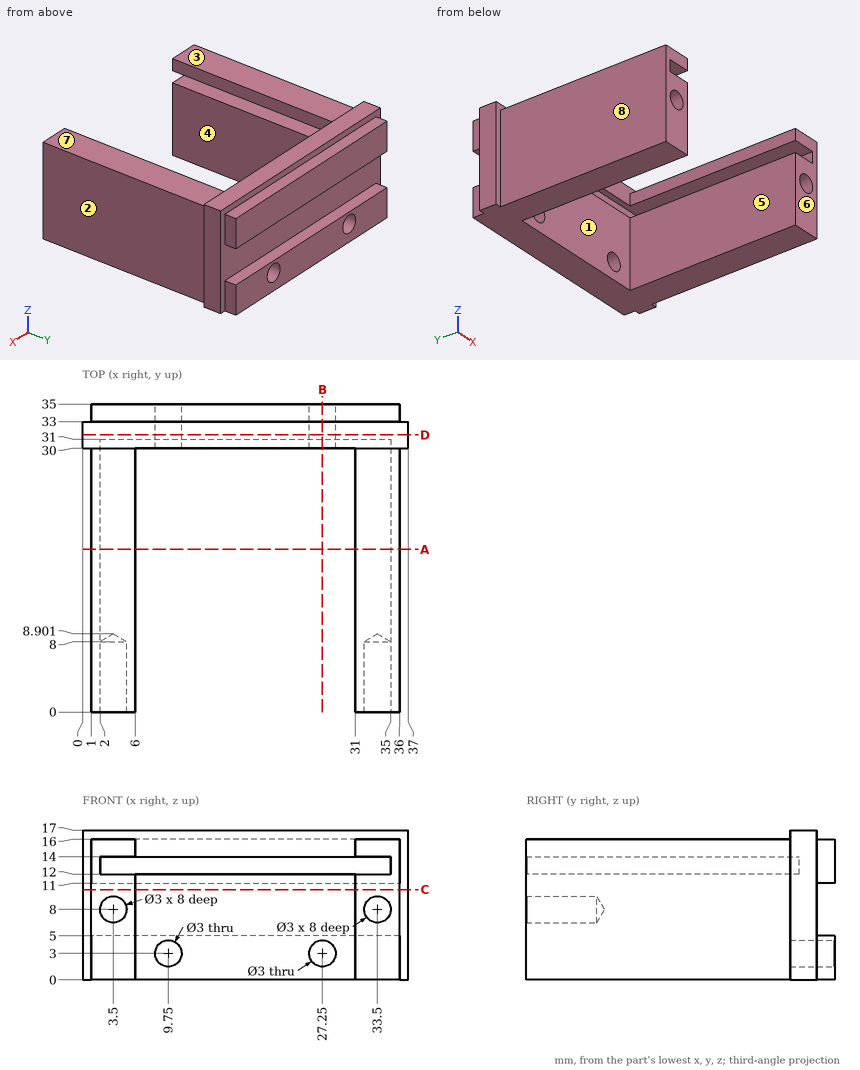
Job drawing, mm, ordinate dimensions from the low corner. One solid piece. A direction names the side the tool comes from. Give positions to 0.01 mm unless a question says otherwise; leave off trailing zeros. Write each loop counter-clockwise with the first axis right and the second up, starting at its lowest first coordinate (ties: lowest second). Pieces come first, ordered by that corner, then holes. Notation, with made-up numbers: (78.25, 28.5) - (116.25, 28.5) arc R16 cw to (116.25, 33.5) - close; hole circle Ø3 at (81.25, 54.5). An arc over 180 degrees is marked (long way). Use one line per item in the form item = value. Start each with the question number.
1. Two-plate mould, pull along X, no slides. Class the marked faces 1, 2, 3 and 4: released by +X, released by -X, zero draft, split by the parting line, or undercut.
2. Band-saw the part on D-D on y = 31.5. Write the cut outline in (x, z).
3. Drop flat-ended pins along their axis: pin 1 Ø1.6 at (y, z) = (34, 12.5) entering from -X; pin 2 Ø1.6 at (x, y) = (17, 34) entering from +Z; pin 3 Ø8 at (x, z) = (16, 14.5) entering from -Y; pin 4 Ø2 at (x, z) = (4, 14) entering from -Y. Give the stop position or say it passes through.
4. Band-saw the part on C-C on z = 10.25. Write the cut outline in (x, y), plus the area to 3 significant figures.
5. Probe line 1 (Z direction, x = 33.5, y = 5); line 2 (Z direction, x = 27.25, y = 33.2); line 3 (X direction, y = 32.2, z = 3). List the from-to ranges inside material, lowest first. Write a range as [from, to].
6. 3-axis set-ups, long thin cutter, end or side, ignore diameter. For the marked faces 5, 6, 7 and 8: which of +Z, -Z, +X, -X, +Y, -Y reach the whole face in a straight line?
7. Band-saw the part on A-A on y = 18.5. Write the cut outline in (x, z), plus the area to 3 significant figures.
8. Band-saw the part on B-B on x = 27.25. Write the cut outline in (y, z).
Conclusion:
q1.face_1 = undercut
q1.face_2 = released by +X
q1.face_3 = zero draft
q1.face_4 = undercut
q2.outline = (0, 0) - (37, 0) - (37, 17) - (0, 17) - close; hole circle Ø3 at (9.75, 3); hole circle Ø3 at (27.25, 3)
q3.pin_1 = 1
q3.pin_2 = 16
q3.pin_3 = 30
q3.pin_4 = 0
q4.outline = (0, 30) - (1, 30) - (1, 0) - (6, 0) - (6, 30) - (31, 30) - (31, 0) - (36, 0) - (36, 30) - (37, 30) - (37, 33) - (0, 33) - close
q4.area = 411 mm²
q5.line_1 = [0, 6.5], [9.5, 12], [14, 16]
q5.line_2 = [0, 1.5], [4.5, 5], [11, 16]
q5.line_3 = [0, 8.25], [11.25, 25.75], [28.75, 37]
q6.face_5 = +Z, -Z, -Y
q6.face_6 = +Z, -Z, +X, -X, -Y
q6.face_7 = +Z, +X, -X, -Y
q6.face_8 = +Z, -Z, -X, -Y
q7.outline = (1, 0) - (6, 0) - (6, 12) - (2, 12) - (2, 14) - (6, 14) - (6, 16) - (1, 16) - close; (31, 0) - (36, 0) - (36, 16) - (31, 16) - (31, 14) - (35, 14) - (35, 12) - (31, 12) - close
q7.area = 144 mm²
q8.outline = (30, 0) - (35, 0) - (35, 1.5) - (30, 1.5) - close; (30, 4.5) - (35, 4.5) - (35, 5) - (33, 5) - (33, 11) - (35, 11) - (35, 16) - (33, 16) - (33, 17) - (30, 17) - (30, 14) - (31, 14) - (31, 12) - (30, 12) - close
